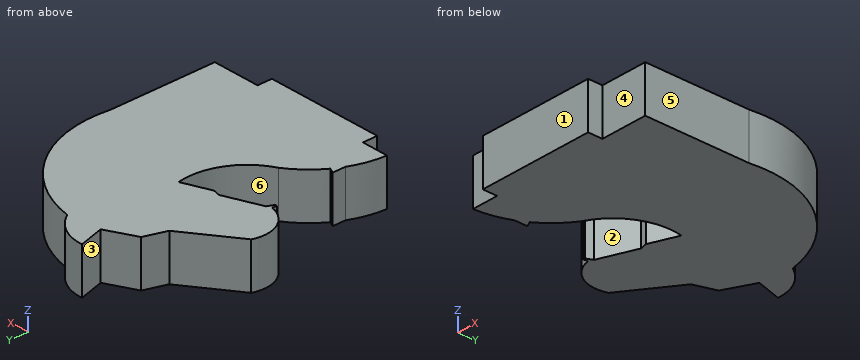
Autodesk Inventor part; units mm, degrees
ref_plane "YZ Plane" through (0, 0, 0) normal (1, 0, 0) x (0, 1, 0)
ref_plane "XZ Plane" through (0, 0, 0) normal (0, 1, 0) x (-1, 0, 0)
ref_plane "XY Plane" through (0, 0, 0) normal (0, 0, 1) x (1, 0, 0)
sketch "Boceto1" plane through (0, 0, 0) normal (0, 0, 1) x (1, 0, 0)
  line L0 (-55.5895, 69.239) -> (57.1029, 69.239) construction
  line L1 (57.1029, 69.239) -> (57.1029, -41.5752) construction
  line L2 (57.1029, -41.5752) -> (-55.5895, -41.5752) construction
  line L3 (-55.5895, -41.5752) -> (-55.5895, 69.239) construction
  line L4 (-12.6216, 0) -> (12.6216, 0)
  line L5 (12.6216, 0) -> (12.6216, 3.1554)
  line L6 (12.6216, 3.1554) -> (22.8766, 3.1554)
  line L7 (22.8766, 3.1554) -> (22.8766, 26.032)
  arc A0 (22.8766, 26.032) -> (2.3665, 54.4304) centre (-1.924, 29.7261) ccw
  arc A1 (2.3665, 54.4304) -> (-6.3108, 59.1635) centre (-5.9164, 49.5659) ccw
  line L8 (-6.3108, 59.1635) -> (-4.7331, 53.6416)
  line L9 (-4.7331, 53.6416) -> (-11.0439, 50.4862)
  line L10 (-11.0439, 50.4862) -> (-12.6216, 45.7531)
  line L11 (-12.6216, 45.7531) -> (-23.6654, 37.8647)
  arc A2 (-23.6654, 37.8647) -> (-18.4064, 28.3985) centre (-16.9879, 35.3805) ccw
  line L12 (-18.4064, 28.3985) -> (-9.4662, 31.9205)
  line L13 (-9.4662, 31.9205) -> (-7.8885, 31.5539)
  line L14 (-7.8885, 31.5539) -> (-1.924, 33.9035)
  arc A3 (-9.4662, 18.8123) -> (-1.924, 33.9035) centre (-15.5194, 31.2678) ccw
  arc A4 (-9.4662, 18.8123) -> (-18.4064, 3.1554) centre (1.3548, 2.2525) ccw
  line L15 (-18.4064, 3.1554) -> (-12.6216, 3.1554)
  line L16 (-12.6216, 3.1554) -> (-12.6216, 0)
  line L17 (-18.4064, 28.3985) -> (-18.4064, 27.4104)
  line L18 (-18.4064, 27.4104) -> (-18.0172, 27.4104)
  line L19 (-18.0172, 27.4104) -> (-17.3546, 28.8128)
  line L20 (-16.5658, 10.6295) -> (-16.5658, 13.4104)
  line L21 (-16.5658, 13.4104) -> (-15.356, 12.8389)
  point P0 (0, 0)
  point P1 (-18.2118, 27.4104)
  dimension "d8" = 14
extrude "Extrusión1" add sketch "Boceto1" along normal mid plane 10
properties part number "KIGTH TOP abrebotella medium 1.1"
Read the model definition and answer for the solid it produces. Units are mm, in the model's axes. Face numbers are marked on the shaded views. A direction names the side the tool comes from. Round coordinates to 2 decimals unless told otherwise and drop trailing zeros. Loops run counter-clockwise (first coordinate to the right, second up) from the corner with the lowest first, then second, coordinate; pieces in that order, holes last.
Q1. Section A-A on y = 30.5 is taken. Write down the section's boundary in (x, z).
Q2. Section D-D on y = 39 is taken. Write down the section's boundary in (x, z), and give its area (3 significant figures).
Q3. Each of these flat-tipped pins is pushed along its axis until it touches: pin 1 (3.5 mm diameter, centred on y = 1.5, z = 0.5, fed in from -X); pin 2 (1.5 mm diameter, centred on y = 17.5, z = 3, fed in from -X); pin 3 (3.5 mm diameter, centred on y = 1, z = 0, fed in from +X). Where does it stop, or does it pass through?
Q4. Which of the six approach directions +Z, -Z, +X, -X, +Y, -Y give full straight-line access (tool end or side, diameter ignored) to the marked faces 1, 2 and 3?
Q5. Section B-B on z = 3.25 is taken. Write down the section's boundary in (x, y), and give its area (3 significant figures).
Q6. Consider probe 1 along Y at (x, z) = (-8.5, 2); probe 2 along X at (y, z) = (12, -1.75); probe 3 along Y at (x, z) = (-16.5, 0.5). Determine where each line is inside the solid, lowest interval first.
Q7. Section C-C on x = 3 is taken. Write down the section's boundary in (y, z).
Q8. Determine the mould class of the marked faces 4, 5 and 6 for opening direction Y: released by +Y, released by -Y, zero draft, split by the parting line, or undercut.
Output:
1. outline: (-22.18, -5) - (-13.07, -5) - (-13.07, 5) - (-22.18, 5) - close; (-1.69, -5) - (23.14, -5) - (23.14, 5) - (-1.69, 5) - close
2. outline: (-22.08, -5) - (21.37, -5) - (21.37, 5) - (-22.08, 5) - close
2. area: 434 mm2
3. pin 1: stops at x = -18.41
3. pin 2: stops at x = -12.1
3. pin 3: stops at x = 12.62
4. face 1: +Z, -Z, +X, -X, -Y
4. face 2: +Z, -Z
4. face 3: +Z, -Z, -X
5. outline: (-23.67, 37.86) arc R7.12 ccw to (-18.41, 28.4) - (-18.41, 27.41) - (-18.02, 27.41) - (-17.35, 28.81) - (-9.47, 31.92) - (-7.89, 31.55) - (-1.92, 33.9) arc R13.85 cw to (-9.47, 18.81) arc R19.78 ccw to (-15.36, 12.84) - (-16.57, 13.41) - (-16.57, 10.63) arc R19.78 ccw to (-18.41, 3.16) - (-12.62, 3.16) - (-12.62, 0) - (12.62, 0) - (12.62, 3.16) - (22.88, 3.16) - (22.88, 26.03) arc R25.07 ccw to (2.37, 54.43) arc R9.61 ccw to (-6.31, 59.16) - (-4.73, 53.64) - (-11.04, 50.49) - (-12.62, 45.75) - close
5. area: 1,850 mm2
6. probe 1: y = 0 to 19.33, 31.7 to 51.76
6. probe 2: x = -16.57 to 22.88
6. probe 3: y = 3.16 to 13.38, 29.15 to 42.98
7. outline: (0, -5) - (54.31, -5) - (54.31, 5) - (0, 5) - close
8. face 4: released by -Y
8. face 5: zero draft
8. face 6: undercut
